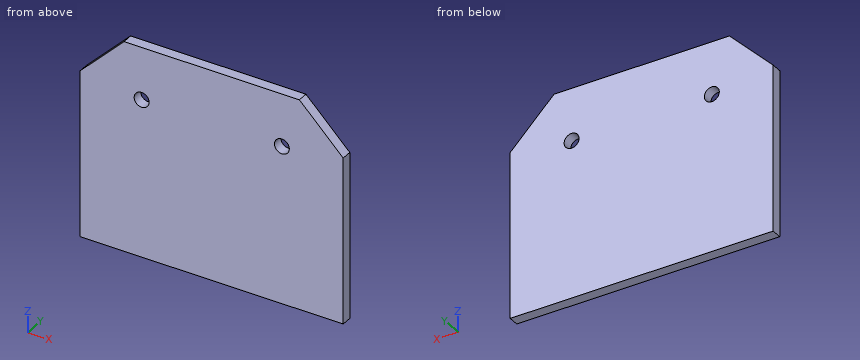
```python
from build123d import *

# Parameters (mm, degrees)
F0_W     = 150
F0_H     = 120
F1_DEPTH = 6
F2_R     = 4.25
F3_DEPTH = 25
F4_SIZE  = 25


with BuildPart() as f1:
    # F0 (on Front) → F1 (new body)
    with BuildSketch(Plane.XZ):
        Rectangle(F0_W, F0_H)
    extrude(amount=F1_DEPTH)

    # F2 (on face) → F3 (cut)
    with BuildSketch(Plane.XZ.offset(6)):
        with Locations((-40, 30)):
            Circle(F2_R)
        with Locations((40, 30)):
            Circle(F2_R)
    extrude(amount=-F3_DEPTH, mode=Mode.SUBTRACT)

    # F4
    f4_edges = [f1.edges().sort_by_distance(p)[0] for p in [
        (-75, -3, 60),
        (75, -3, 60),
    ]]
    chamfer(f4_edges, length=F4_SIZE)


solid = f1.part
```
Geometry check sheet. Reference: the model listing, model coordinates, mm. Give positions to 0.01 mm unless a question says otherwise; leave off trailing zeros. Loops run counter-clockwise (first coordinate to the right, second up) from the corner with the lowest first, then second, coordinate; pieces in that order, holes last. Notation, with made-up numbers: M 73,84.5 L 119,84.5 A19 cw 119,109.5 Z; hole C 14.25,80 d4. An arc over 180 degrees is marked long. Write item = value, one per line.
(1) Sectioned sample at D-D, the plane x = -57.5. Record the cut outline in (y, z).
Answer below:
outline = M -6,-60 L 0,-60 L 0,52.5 L -6,52.5 Z
(2) Material ranges on line 1 (Z direction, x = 40, y = -2.95); line 2 (X direction, y = -3.5, z = 28.5); line 3 (Z direction, x = 41, y = -1.5), recorded low to high. Write a range as [from, to].
Answer below:
line_1 = [-60, 25.75], [34.25, 60]
line_2 = [-75, -43.98], [-36.02, 36.02], [43.98, 75]
line_3 = [-60, 25.87], [34.13, 60]
(3) Gauge pin test, flat end, axial feed: pin 1 Ø5 at (x, z) = (40, 30) entering from +Y. Record the tip position at first contact, or that the pin passes through.
Answer below:
pin_1 = through
(4) Sectioned sample at A-A, the plane z = 30. Record the cut outline in (x, y).
Answer below:
outline = M -75,-6 L -44.25,-6 L -44.25,0 L -75,0 Z; M -35.75,-6 L 35.75,-6 L 35.75,0 L -35.75,0 Z; M 44.25,-6 L 75,-6 L 75,0 L 44.25,0 Z
(5) Sectioned sample at C-C, the plane y = -3.75. Record the cut outline in (x, z).
Answer below:
outline = M -75,-60 L 75,-60 L 75,35 L 50,60 L -50,60 L -75,35 Z; hole C -40,30 d8.5; hole C 40,30 d8.5
(6) Sectioned sample at B-B, the plane x = 40. Record the cut outline in (y, z), plus the area to 3 significant figures.
Answer below:
outline = M -6,-60 L 0,-60 L 0,25.75 L -6,25.75 Z; M -6,34.25 L 0,34.25 L 0,60 L -6,60 Z
area = 669 mm2
